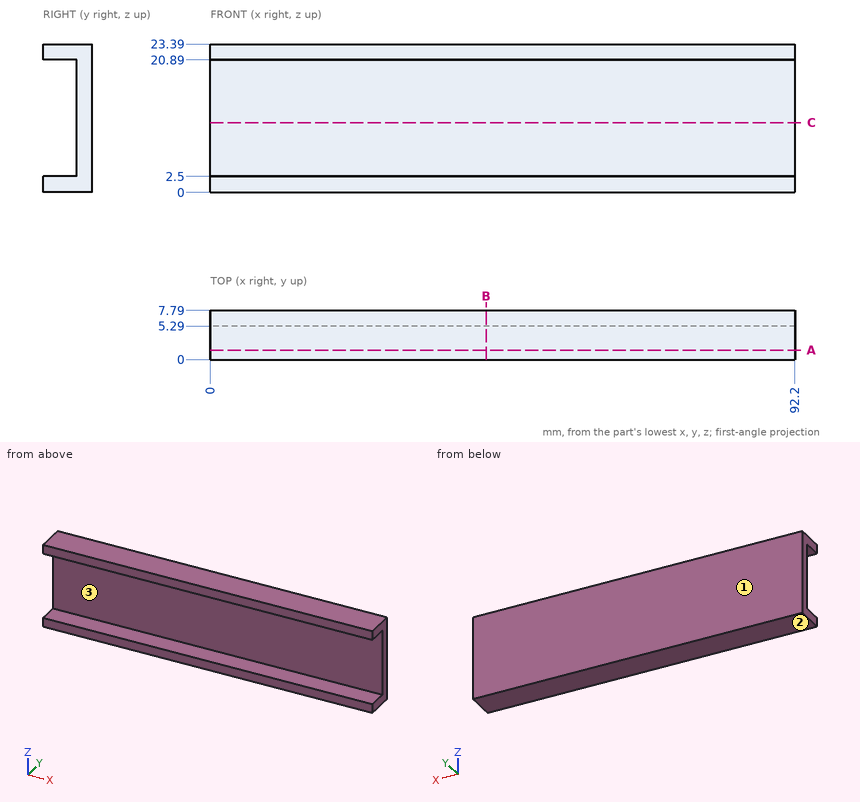
Can you work these out from the drawing? Everything is in mm from the part's minimum corner. Give positions to 0.01 mm unless a question says otherwise; leave off trailing zeros. Loops run counter-clockwise (first coordinate to the right, second up) from the corner with the lowest first, then second, coordinate; pieces in that order, holes last. Notation, with made-up numbers: (50.25, 7.5) -> (61.25, 7.5) arc R14 ccw to (61.25, 28.5) -> close; hole circle Ø1 at (44.25, 25). An arc over 180 degrees is marked (long way). Return JSON: item names as keys, results as strings.
Item 1: If we section it at C-C on z = 11: List the corners of the cut face in (x, y) for me, plus the area to 4 significant figures.
Geometry results:
{"outline": "(0, 5.29) -> (92.2, 5.29) -> (92.2, 7.79) -> (0, 7.79) -> close", "area": "230.5 mm²"}
Item 2: I'm going to push flat-ended pins straight in: pin 1 (6 mm diameter, centred on x = 72, z = 10.5, fed in from -Y); pin 2 (4 mm diameter, centred on y = 2.5, z = 17.5, fed in from +X). Where does each tip first touch, or does it pass through?
Geometry results:
{"pin 1": "stops at y = 5.29", "pin 2": "passes through"}
Item 3: I need wall thicknesses on L1, parallel to Z at x = 49, y = 5.25; L2, parallel to Y at x = 36.5, z = 17. Which ranges of each line are inside material? Lowest first, please. Write a range as from..to.
Geometry results:
{"L1": "z = 0..2.5, 20.89..23.39", "L2": "y = 5.29..7.79"}
Item 4: We'd pull the mould along Z, two halves only. Please class the marked faces 1, 2 and 3: +Z half, -Z half, draft (parallel to the pull), parting line (faces both ways), or undercut.
Geometry results:
{"face 1": "draft", "face 2": "-Z half", "face 3": "undercut"}
Item 5: If we section it at A-A on y = 1.5: List the corners of the cut face in (x, z) for me, plus the area to 3 significant figures.
Geometry results:
{"outline": "(0, 0) -> (92.2, 0) -> (92.2, 2.5) -> (0, 2.5) -> close; (0, 20.89) -> (92.2, 20.89) -> (92.2, 23.39) -> (0, 23.39) -> close", "area": "461 mm²"}
Item 6: If we section it at B-B on x = 43.5: List the corners of the cut face in (y, z) for me.
Geometry results:
{"outline": "(0, 0) -> (7.79, 0) -> (7.79, 23.39) -> (0, 23.39) -> (0, 20.89) -> (5.29, 20.89) -> (5.29, 2.5) -> (0, 2.5) -> close"}
